from build123d import *

# Parameters (mm, degrees)
SKETCH1_W                = 32
SKETCH1_H                = 29
BOSS_EXTRUDE1_DEPTH      = 35
FILLET1_R                = 2
SLOT_FOR_COIL_DEPTH      = 1
SLOT_FOR_COIL_DEPTH_BACK = 30
BOSS_EXTRUDE2_DEPTH      = 7
BOSS_EXTRUDE3_DEPTH      = 1.75
SKETCH5_W                = 2
SKETCH5_H                = 7
CUT_EXTRUDE2_DEPTH       = 33
CUT_EXTRUDE3_DEPTH       = 22
SKETCH7_W                = 2
SKETCH7_H                = 33
BOSS_EXTRUDE4_DEPTH      = 0.25
FILLET2_R                = 6
CUT_EXTRUDE5_DEPTH       = 4.5
SKETCH14_W               = 2.5
SKETCH14_H               = 20
CUT_EXTRUDE6_DEPTH       = 22
SKETCH16_W               = 2
SKETCH16_H               = 2
BOSS_EXTRUDE5_DEPTH      = 22
BOSS_EXTRUDE6_DEPTH      = 22
SKETCH21_W               = 10
SKETCH21_H               = 2
BOSS_EXTRUDE7_DEPTH      = 2.5
SKETCH23_W               = 8
SKETCH23_H               = 1.5
CUT_EXTRUDE7_DEPTH       = 2
FILLET3_R                = 1
CUT_EXTRUDE8_REACH       = 34
SKETCH26_R               = 5


with BuildPart() as part:
    # Sketch1 → Boss-Extrude1 (new body)
    with BuildSketch(Plane.XY):
        Rectangle(SKETCH1_W, SKETCH1_H)
    extrude(amount=BOSS_EXTRUDE1_DEPTH)

    # Fillet1
    fillet1_edges = [part.edges().sort_by_distance(p)[0] for p in [
        (16, -14.5, 17.5),
        (-16, -14.5, 17.5),
        (-16, 14.5, 17.5),
        (16, 14.5, 17.5),
    ]]
    fillet(fillet1_edges, radius=FILLET1_R)

    # Sketch2 → Slot for Coil (cut, two sides)
    with BuildSketch(Plane.XZ.offset(14.5)) as slot_for_coil_sk:
        Polygon((-9.125, 0), (-9.125, 1.75), (-11.125, 1.75), (-11.125, 5), (11.125, 5), (11.125, 1.75), (9.125, 1.75), (9.125, 0), align=None)
    extrude(amount=SLOT_FOR_COIL_DEPTH, mode=Mode.SUBTRACT)
    extrude(slot_for_coil_sk.sketch, amount=-SLOT_FOR_COIL_DEPTH_BACK, mode=Mode.SUBTRACT)

    # Sketch3 → Boss-Extrude2 (add)
    with BuildSketch(Plane.XZ.offset(14.5)):
        Polygon((-9.125, 0), (-9.125, 1.75), (-11.125, 1.75), (-11.125, 5), (11.125, 5), (11.125, 1.75), (9.125, 1.75), (9.125, 0), align=None)
    extrude(amount=-BOSS_EXTRUDE2_DEPTH)

    # Sketch4 → Boss-Extrude3 (add)
    with BuildSketch(Plane(origin=(0, 0, 1.75), x_dir=(-1, 0, 0), z_dir=(0, 0, -1))):
        with BuildLine():
            Line((-9.125, 7.5), (-9.125, 6.5))
            ThreePointArc((-9.125, 6.5), (-8.875, 7), (-9.125, 7.5))
        make_face()
    boss_extrude3 = extrude(amount=BOSS_EXTRUDE3_DEPTH)

    # Mirror1: Boss-Extrude3 across plane
    add(boss_extrude3.mirror(Plane(origin=(0, 0, 0), x_dir=(0, 0, 1), z_dir=(1, 0, 0))))

    # Sketch5 → Cut-Extrude2 (cut)
    with BuildSketch(Plane(origin=(0, 0, 0), x_dir=(-1, 0, 0), z_dir=(0, 0, -1))):
        with Locations((0, -11)):
            Rectangle(SKETCH5_W, SKETCH5_H)
    extrude(amount=-CUT_EXTRUDE2_DEPTH, mode=Mode.SUBTRACT)

    # Sketch6 → Cut-Extrude3 (cut)
    with BuildSketch(Plane(origin=(0, 14.5, 0), x_dir=(1, 0, 0), z_dir=(0, 1, 0))):
        Polygon((-12.5, -7.5), (-12.5, -11), (-11.5, -11), (-11.5, -33), (11.5, -33), (11.5, -11), (12.5, -11), (12.5, -7.5), align=None)
    extrude(amount=-CUT_EXTRUDE3_DEPTH, mode=Mode.SUBTRACT)

    # Sketch7 → Boss-Extrude4 (add)
    with BuildSketch(Plane.XZ.offset(14.5)):
        with Locations((0, 16.5)):
            Rectangle(SKETCH7_W, SKETCH7_H)
    extrude(amount=-BOSS_EXTRUDE4_DEPTH)

    # Fillet2
    fillet2_edges = [part.edges().sort_by_distance(p)[0] for p in [
        (0, -14.25, 33),
    ]]
    fillet(fillet2_edges, radius=FILLET2_R)

    # Sketch11 → Cut-Extrude5 (cut)
    with BuildSketch(Plane(origin=(-16, 0, 44), x_dir=(0, 0, -1), z_dir=(1, 0, 0))):
        with BuildLine():
            Line((24.25, 25), (24.25, 0))
            ThreePointArc((24.25, 0), (21, -3.25), (17.75, 0))
            Line((17.75, 0), (17.75, 25))
            ThreePointArc((17.75, 25), (21, 28.25), (24.25, 25))
        make_face()
    extrude(amount=CUT_EXTRUDE5_DEPTH, mode=Mode.SUBTRACT)

    # Sketch14 → Cut-Extrude6 (cut)
    with BuildSketch(Plane(origin=(0, 14.5, 0), x_dir=(1, 0, 0), z_dir=(0, 1, 0))):
        with Locations((-12.75, -23)):
            Rectangle(SKETCH14_W, SKETCH14_H)
    extrude(amount=-CUT_EXTRUDE6_DEPTH, mode=Mode.SUBTRACT)

    # Sketch16 → Boss-Extrude5 (add)
    with BuildSketch(Plane(origin=(0, 14.5, 0), x_dir=(1, 0, 0), z_dir=(0, 1, 0))):
        with Locations((-11, -14)):
            Rectangle(SKETCH16_W, SKETCH16_H)
        with Locations((-11, -32)):
            Rectangle(SKETCH16_W, SKETCH16_H)
    extrude(amount=-BOSS_EXTRUDE5_DEPTH)

    # Sketch20 → Boss-Extrude6 (add)
    with BuildSketch(Plane(origin=(0, 14.5, 0), x_dir=(1, 0, 0), z_dir=(0, 1, 0))):
        Polygon((-11.5, -11), (-10, -13), (-11.5, -13), align=None)
        Polygon((-10, -31), (-8.5, -33), (-10, -33), align=None)
    extrude(amount=-BOSS_EXTRUDE6_DEPTH)

    # Sketch21 → Boss-Extrude7 (add)
    with BuildSketch(Plane(origin=(0, 14.5, 0), x_dir=(-1, 0, 0), z_dir=(0, 1, 0))):
        with Locations((0, 34)):
            Rectangle(SKETCH21_W, SKETCH21_H)
    boss_extrude7 = extrude(amount=BOSS_EXTRUDE7_DEPTH)

    # Sketch23 → Cut-Extrude7 (cut)
    with BuildSketch(Plane.XY.offset(35)):
        with Locations((0, 15.75)):
            Rectangle(SKETCH23_W, SKETCH23_H)
    cut_extrude7 = extrude(amount=-CUT_EXTRUDE7_DEPTH, mode=Mode.SUBTRACT)

    # Mirror3: Boss-Extrude7, Cut-Extrude7 across plane
    add(boss_extrude7.mirror(Plane.ZX))
    add(cut_extrude7.mirror(Plane.ZX), mode=Mode.SUBTRACT)

    # Fillet3
    fillet3_edges = [part.edges().sort_by_distance(p)[0] for p in [
        (5, 14.5, 34),
        (-5, 14.5, 34),
        (5, 17, 34),
        (-5, 17, 34),
        (5, -17, 34),
        (-5, -17, 34),
        (5, -14.5, 34),
        (-5, -14.5, 34),
    ]]
    fillet(fillet3_edges, radius=FILLET3_R)

    # Sketch26 → Cut-Extrude8 (cut, up to next)
    with BuildSketch(Plane(origin=(16, 0, 0), x_dir=(0, 0, -1), z_dir=(1, 0, 0)), mode=Mode.PRIVATE) as cut_extrude8_sk1:
        with Locations((-17.485, -2.89)):
            Circle(SKETCH26_R)
    cut_extrude8_tool1 = extrude(cut_extrude8_sk1.sketch, amount=-CUT_EXTRUDE8_REACH, mode=Mode.PRIVATE) & part.part
    add(cut_extrude8_tool1.solids().sort_by_distance((16, -2.89, 17.485))[0], mode=Mode.SUBTRACT)


solid = part.part
Here's how the part is built. I have some questions about the finished solid (model axes, mm). A direction names the side the tool comes from. Give positions to 0.01 mm unless a question says otherwise; leave off trailing zeros. Loops run counter-clockwise (first coordinate to the right, second up) from the corner with the lowest first, then second, coordinate; pieces in that order, holes last. Notation, with made-up numbers: (18, 55.25) -> (28, 55.25) arc R15 ccw to (28, 73.25) -> close; hole circle Ø4 at (-19.75, 24.5). An arc over 180 degrees is marked (long way). One line per item, written item: value.
Q1. On a 3-axis mill with a long thin cutter (end or side, diameter ignored), from which of +Z, -Z, +X, -X, +Y, -Y can I reach the whole of each face in a straight line? I mean faces 1 (the face through (-16, 0, 17)), 2 (the face through (-13, 4, 33)), 3 (the face through (11.94, -7.77, 18.57)). Say none if no direction works.
Answers follow:
face 1: +Z, -Z, -X, +Y, -Y
face 2: +Y
face 3: +X
Q2. Suppose I cut it at C-C on x = 8. Please give me the cut outline in (y, z) (3 decimals), then the cut area to 3 significant figures.
Answers follow:
outline: (-14.5, 0) -> (-7.5, 0) -> (-7.5, 5) -> (14.5, 5) -> (14.5, 7.5) -> (-7.5, 7.5) -> (-7.5, 15.549) arc R5 cw to (-7.5, 19.421) -> (-7.5, 33) -> (14.5, 33) -> (14.5, 35) -> (-14.5, 35) -> close
area: 343 mm^2
Q3. We'd pull the mould along X, two halves only. Please class faces 4 (the face through (16, 3, 17)), 5 (the face through (-9.26, 3.654, 31.986)), 6 (the face through (-15.43, -13.9, 17.74)): pulls with the +X half, pulls with the -X half, needs draft (parallel to the pull), parting line crosses it, or undercut.
Answers follow:
face 4: pulls with the +X half
face 5: undercut
face 6: pulls with the -X half
Q4. If I drill on line 1 along Z through (x, y) = (11, -2); line 2 along X through (y, z) = (8, 15.5); line 3 along X through (y, z) = (-12.5, 6.5), over which ranges is the centre line in solid material (lowest first)?
Answers follow:
line 1: 0 to 1.75, 5 to 7.5, 33 to 35
line 2: -16 to -14, 11.5 to 16
line 3: -16 to -1, 1 to 16
Q5. Suppose I cut it at D-D on z = 14. Please give me the cut outline in (x, y), then the cut area to 3 significant figures.
Answers follow:
outline: (-16, -12.5) arc R2 ccw to (-14, -14.5) -> (14, -14.5) arc R2 ccw to (16, -12.5) -> (16, -6.48) -> (11.5, -6.48) -> (11.5, -7.5) -> (1, -7.5) -> (1, -14.25) -> (-1, -14.25) -> (-1, -7.5) -> (-10, -7.5) -> (-10, 14.5) -> (-12, 14.5) -> (-12, -7.5) -> (-14, -7.5) -> (-14, 14.5) arc R2 ccw to (-16, 12.5) -> close; (11.5, 0.7) -> (16, 0.7) -> (16, 12.5) arc R2 ccw to (14, 14.5) -> (11.5, 14.5) -> close
area: 362 mm^2
Q6. Suppose I cut it at A-A on z = 23. Please give me the cut outline in (x, y), then the cut area to 3 significant figures.
Answers follow:
outline: (-16, -12.5) arc R2 ccw to (-14, -14.5) -> (14, -14.5) arc R2 ccw to (16, -12.5) -> (16, 12.5) arc R2 ccw to (14, 14.5) -> (11.5, 14.5) -> (11.5, -7.5) -> (1, -7.5) -> (1, -14.25) -> (-1, -14.25) -> (-1, -7.5) -> (-14, -7.5) -> (-14, -3.25) -> (-16, -3.25) -> close
area: 315 mm^2
Q7. I'm going to push flat-ended pins straight in: pin 1 Ø1 at (x, z) = (0.5, 6.5) entering from -Y; pin 2 Ø1.2 at (y, z) = (-16, 33.5) entering from -X (3 decimals); pin 3 Ø0.6 at (x, z) = (0.5, 11) entering from +Y. Where does each tip first touch, or does it pass through?
Answers follow:
pin 1: y = -14.5
pin 2: x = -5.005
pin 3: y = -14.25
